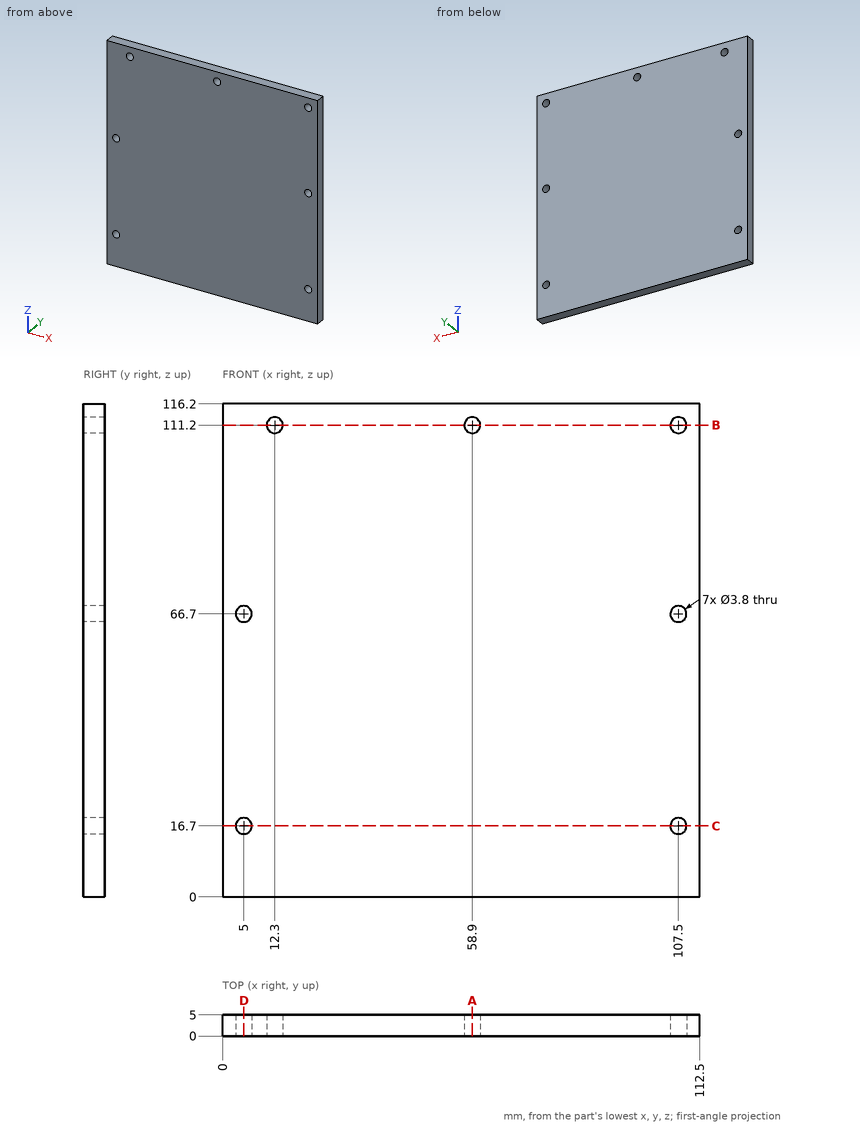
Check sheet for the drawn part. Datum: minimum x, y, z corner. Units: mm. Coordinates: 2 decimals unless noted, no trailing zeros. Order: outer loops, then holes, each group sorted by start corner. A loop starts at its lowest first (then second) coordinate and runs counter-clockwise, first axis right, second up. Notation, with made-up numbers: (-17.75, 26) - (40.25, 26) arc R23 ccw to (40.25, 40) - close; hole circle Ø9 at (88.5, 57.5). An arc over 180 degrees is marked (long way). Return JSON: item names as keys, results as strings.
(1) Section check A-A, the plane x = 58.9. Record the cut outline in (y, z).
Filled sheet:
{"outline": "(0, 0) - (5, 0) - (5, 109.3) - (0, 109.3) - close; (0, 113.1) - (5, 113.1) - (5, 116.2) - (0, 116.2) - close"}
(2) Thickness scan on line 1 along X through (y, z) = (3.95, 111.2); line 2 along X through (y, z) = (2.9, 16.7); line 3 along Z through (x, y) = (5, 2.9). Record the ranges inside material, lowest first.
Filled sheet:
{"line 1": "x = 0 to 10.4, 14.2 to 57, 60.8 to 105.6, 109.4 to 112.5", "line 2": "x = 0 to 3.1, 6.9 to 105.6, 109.4 to 112.5", "line 3": "z = 0 to 14.8, 18.6 to 64.8, 68.6 to 116.2"}
(3) Section check B-B, the plane z = 111.2. Record the cut outline in (x, y), and give its area (4 significant figures).
Filled sheet:
{"outline": "(0, 0) - (10.4, 0) - (10.4, 5) - (0, 5) - close; (14.2, 0) - (57, 0) - (57, 5) - (14.2, 5) - close; (60.8, 0) - (105.6, 0) - (105.6, 5) - (60.8, 5) - close; (109.4, 0) - (112.5, 0) - (112.5, 5) - (109.4, 5) - close", "area": "505.5 mm^2"}
(4) Go/stop test with a flat-tipped pin: pin 1 (3.5 mm diameter, centred on x = 107.5, z = 111.2, fed in from +Y) (3 decimals). Record where the tip stops, or that it passes through.
Filled sheet:
{"pin 1": "passes through"}
(5) Section check D-D, the plane x = 5. Record the cut outline in (y, z).
Filled sheet:
{"outline": "(0, 0) - (5, 0) - (5, 14.8) - (0, 14.8) - close; (0, 18.6) - (5, 18.6) - (5, 64.8) - (0, 64.8) - close; (0, 68.6) - (5, 68.6) - (5, 116.2) - (0, 116.2) - close"}
(6) Section check C-C, the plane z = 16.7. Record the cut outline in (x, y), and give its area (4 significant figures).
Filled sheet:
{"outline": "(0, 0) - (3.1, 0) - (3.1, 5) - (0, 5) - close; (6.9, 0) - (105.6, 0) - (105.6, 5) - (6.9, 5) - close; (109.4, 0) - (112.5, 0) - (112.5, 5) - (109.4, 5) - close", "area": "524.5 mm^2"}
